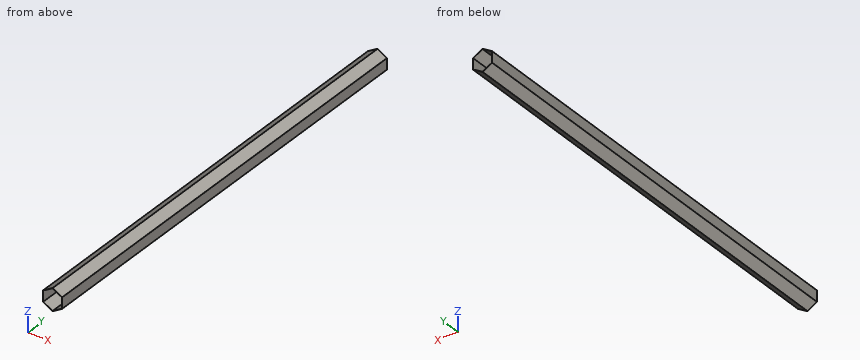
Autodesk Inventor part; units mm, degrees
ref_plane "YZ Plane" through (0, 0, 0) normal (1, 0, 0) x (0, 1, 0)
ref_plane "XZ Plane" through (0, 0, 0) normal (0, 1, 0) x (-1, 0, 0)
ref_plane "XY Plane" through (0, 0, 0) normal (0, 0, 1) x (1, 0, 0)
sketch "Sketch1" plane through (0, 0, 0) normal (0, 1, 0) x (-1, 0, 0)
  line L0 (-2.5, 1.4434) -> (0, 2.8868)
  line L1 (0, 2.8868) -> (2.5, 1.4434)
  line L2 (2.5, 1.4434) -> (2.5, -1.4434)
  line L3 (2.5, -1.4434) -> (0, -2.8868)
  line L4 (0, -2.8868) -> (-2.5, -1.4434)
  line L5 (-2.5, -1.4434) -> (-2.5, 1.4434)
  line L6 (-2.45, 1.4145) -> (0, 2.829)
  line L7 (0, 2.829) -> (2.45, 1.4145)
  line L8 (2.45, 1.4145) -> (2.45, -1.4145)
  line L9 (2.45, -1.4145) -> (0, -2.829)
  line L10 (0, -2.829) -> (-2.45, -1.4145)
  line L11 (-2.45, -1.4145) -> (-2.45, 1.4145)
  point P0 (0, 0)
  point P1 (0, 0)
  point P2 (0, 0)
  dimension "d0" = 5
  dimension "d1" = 4.9
extrude "Extrusion1" add sketch "Sketch1" along normal blind 120
fillet "Fillet1" radius 0.1 6 edges at (0, 60, 2.8868) (2.5, 60, -1.4434) (0, 60, -2.8868) (-2.5, 60, -1.4434) (-2.5, 60, 1.4434) (2.5, 60, 1.4434)
properties part number "Pencil Outside"
Work out the finished part from the listing and answer in its coordinate system (mm). Give positions to 0.01 mm unless a question says otherwise; leave off trailing zeros. Loops run counter-clockwise (first coordinate to the right, second up) from the corner with the lowest first, then second, coordinate; pieces in that order, holes last. Notation, with made-up numbers: (-18.75, 14) - (18.25, 14) arc R16 ccw to (18.25, 39) - close; hole circle Ø8 at (-25, -18). An arc over 180 degrees is marked (long way). Answer in a Markdown table with one row per item. Add a question column.
Q1. The part is cut by section C-C (x = -1.6). Determine the outline of the cut face in (y, z), and give its area (3 significant figures).
Q2. This flat-tipped pin is pushed along its axis until it touches: P1, Ø3, axis at x = 2, y = 41.5, coming from the -Z side. Where does it stop, or does it pass through?
Q3. The part is cut by section A-A (z = 0.35). Determine the outline of the cut face in (x, y), and give its area (3 significant figures).
Q4. The part is cut by section B-B (y = 26). Determine the outline of the cut face in (x, z), and give its area (3 significant figures).
Solution:
| question | item | result |
|---|---|---|
| 1 | outline | (0, -1.96) - (120, -1.96) - (120, -1.91) - (0, -1.91) - close; (0, 1.91) - (120, 1.91) - (120, 1.96) - (0, 1.96) - close |
| 1 | area | 13.9 mm² |
| 2 | P1 | stops at z = -2.6 |
| 3 | outline | (-2.5, 0) - (-2.45, 0) - (-2.45, 120) - (-2.5, 120) - close; (2.45, 0) - (2.5, 0) - (2.5, 120) - (2.45, 120) - close |
| 3 | area | 12.0 mm² |
| 4 | outline | (-2.5, -1.39) arc R0.1 ccw to (-2.45, -1.47) - (-0.05, -2.86) arc R0.1 ccw to (0.05, -2.86) - (2.45, -1.47) arc R0.1 ccw to (2.5, -1.39) - (2.5, 1.39) arc R0.1 ccw to (2.45, 1.47) - (0.05, 2.86) arc R0.1 ccw to (-0.05, 2.86) - (-2.45, 1.47) arc R0.1 ccw to (-2.5, 1.39) - close; hole (-2.45, -1.41) - (0, -2.83) - (2.45, -1.41) - (2.45, 1.41) - (0, 2.83) - (-2.45, 1.41) - close |
| 4 | area | 0.855 mm² |
